from build123d import *

# Parameters (mm, degrees)
SKETCH1_W           = 3.5
SKETCH1_H           = 3.5
BOSS_EXTRUDE1_DEPTH = 1.81
SKETCH2_W           = 0.5
SKETCH2_H           = 0.5
BOSS_EXTRUDE2_DEPTH = 3
SKETCH6_R           = 1
CUT_EXTRUDE1_DEPTH  = 0.001
SKETCH7_R           = 1.2
BOSS_EXTRUDE6_DEPTH = 2.69
HOLE1_D             = 1.6
HOLE1_DEPTH         = 1.45
CHAMFER3_SIZE       = 0.15
SKETCH12_R          = 0.381
BOSS_EXTRUDE7_DEPTH = 3.001
CHAMFER1_SIZE       = 0.15
CHAMFER2_SIZE       = 0.35
CHAMFER2_SIZE2      = 0.15


with BuildPart() as part:
    # Sketch1 → Boss-Extrude1 (new body)
    with BuildSketch(Plane.XZ):
        Rectangle(SKETCH1_W, SKETCH1_H)
    extrude(amount=-BOSS_EXTRUDE1_DEPTH)

    # Sketch2 → Boss-Extrude2 (add)
    with BuildSketch(Plane.XZ):
        with Locations((-1.27, -1.27)):
            Rectangle(SKETCH2_W, SKETCH2_H)
        with Locations((1.27, -1.27)):
            Rectangle(SKETCH2_W, SKETCH2_H)
        with Locations((1.27, 1.27)):
            Rectangle(SKETCH2_W, SKETCH2_H)
        with Locations((-1.27, 1.27)):
            Rectangle(SKETCH2_W, SKETCH2_H)
    extrude(amount=BOSS_EXTRUDE2_DEPTH)

    # Sketch6 → Cut-Extrude1 (cut)
    with BuildSketch(Plane.XZ):
        with Locations(Location((0, 0, 0), (0, 0, 90))):
            Circle(SKETCH6_R)
    extrude(amount=-CUT_EXTRUDE1_DEPTH, mode=Mode.SUBTRACT)

    # Sketch7 → Boss-Extrude6 (add)
    with BuildSketch(Plane(origin=(0, 1.81, 0), x_dir=(-1, 0, 0), z_dir=(0, 1, 0))):
        with Locations(Location((0, 0, 0), (0, 0, 270))):
            Circle(SKETCH7_R)
    extrude(amount=BOSS_EXTRUDE6_DEPTH)

    # Hole1
    with Locations(Plane(origin=(0, 4.5, 0), x_dir=(1, 0, 0), z_dir=(0, 1, 0))):
        with Locations((0, 0)):
            Hole(HOLE1_D / 2, depth=HOLE1_DEPTH)

    # Sketch10 → Revolve1 (revolve)
    with BuildSketch(Plane(origin=(0, 0, 0), x_dir=(-1, 0, 0), z_dir=(0, 0, -1)), mode=Mode.PRIVATE) as revolve1_sk:
        Polygon((-0.19, 3.05), (0, 3.05), (0, 4.37), (-0.0405, 4.37), (-0.19, 4.37), (-0.19, 4.220000833), align=None)
    revolve(revolve1_sk.sketch.rotate(Axis((0, 3.05, 0), (0, 1, 0)), 270), axis=Axis((0, 3.05, 0), (0, 1, 0)))

    # Chamfer3
    chamfer3_edges = [part.edges().sort_by_distance(p)[0] for p in [
        (0, 4.37, -0.19),
    ]]
    chamfer(chamfer3_edges, length=CHAMFER3_SIZE)

    # Sketch12 → Boss-Extrude7 (add)
    with BuildSketch(Plane.XZ.offset(-0.001)):
        with Locations(Location((0, 0, 0), (0, 0, 90))):
            Circle(SKETCH12_R)
    extrude(amount=BOSS_EXTRUDE7_DEPTH)

    # Chamfer1
    chamfer1_edges = [part.edges().sort_by_distance(p)[0] for p in [
        (0, -3, -0.381),
    ]]
    chamfer(chamfer1_edges, length=CHAMFER1_SIZE)

    # Chamfer2
    chamfer2_edges = [part.edges().sort_by_distance(p)[0] for p in [
        (0, 4.5, 1.2),
    ]]
    chamfer2_side = [part.faces().sort_by_distance(p)[0] for p in [
        (0, 3.155, 1.2),
    ]]
    chamfer(chamfer2_edges, length=CHAMFER2_SIZE, length2=CHAMFER2_SIZE2, reference=chamfer2_side[0])


solid = part.part
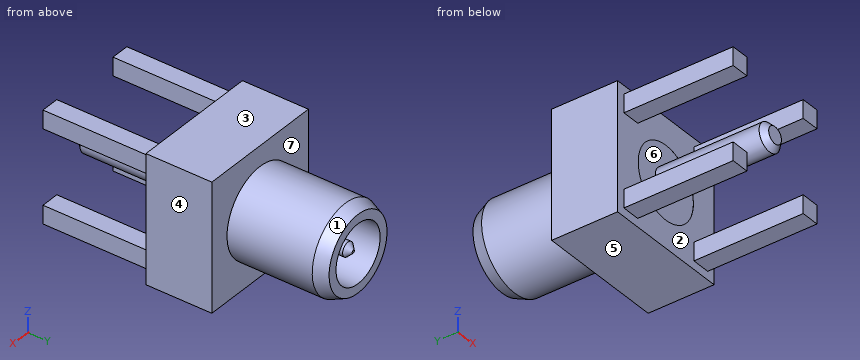
Part model, mm, in its own coordinate system. Face numbers are marked on the shaded views. A direction names the side the tool comes from. Coordinates: 2 decimals unless noted, no trailing zeros. Write each loop counter-clockwise with the first axis right and the second up, starting at its lowest first coordinate (ties: lowest second). Pieces come first, ordered by that corner, then holes. Notation, with made-up numbers: (82.5, 28) - (130.5, 28) arc R25 ccw to (130.5, 65) - close; hole circle Ø9 at (1.5, -24). An arc over 180 degrees is marked (long way). Put each result on its own line as item: value.
1. Probe line 1 along X through (y, z) = (-1.5, 1.4); line 2 along Y through (x, z) = (0.05, 0.65); line 3 along Y through (x, z) = (1.4, 0.45). List the from-to ranges inside material, lowest first. Write a range as [from, to].
Final values:
line 1: x = [-1.52, -1.02], [1.02, 1.52]
line 2: y = [0, 3.05]
line 3: y = [0, 1.81]
2. 3-axis set-ups, long thin cutter, end or side, ignore diameter. For the marked faces 5, 6 and 7: which of +Z, -Z, +X, -X, +Y, -Y reach the whole face in a straight line?
Final values:
face 5: -Z, +X, -X, +Y, -Y
face 6: -Y
face 7: +Y
3. Flat gauge pins, fed straight in: pin 1 Ø0.6 at (x, y) = (-1.5, -1.5) entering from -Z; pin 2 Ø2 at (x, y) = (1, -1.5) entering from +Z; pin 3 Ø0.6 at (y, z) = (-1.5, -1.5) entering from -X. Where does each tip first touch, or does it go through?
Final values:
pin 1: stops at z = -1.52
pin 2: stops at z = 1.52
pin 3: stops at x = -1.52
4. Band-saw the part on B-B (y = -1). Write the cut outline in (x, z), then the cut area to 3 significant figures.
Final values:
outline: (-1.52, -1.52) - (-1.02, -1.52) - (-1.02, -1.02) - (-1.52, -1.02) - close; (-1.52, 1.02) - (-1.02, 1.02) - (-1.02, 1.52) - (-1.52, 1.52) - close; circle Ø0.76 at (0, 0); (1.02, -1.52) - (1.52, -1.52) - (1.52, -1.02) - (1.02, -1.02) - close; (1.02, 1.02) - (1.52, 1.02) - (1.52, 1.52) - (1.02, 1.52) - close
area: 1.46 mm²
5. Band-saw the part on C-C (z = 1.4). Write the cut outline in (x, y), then the cut area to 4 significant figures.
Final values:
outline: (-1.75, 0) - (-1.52, 0) - (-1.52, -3) - (-1.02, -3) - (-1.02, 0) - (1.02, 0) - (1.02, -3) - (1.52, -3) - (1.52, 0) - (1.75, 0) - (1.75, 1.81) - (-1.75, 1.81) - close
area: 9.335 mm²
6. Band-saw the part on D-D (x = 1.3). Write the cut outline in (y, z), then the cut area to 4 significant figures.
Final values:
outline: (-3, -1.52) - (0, -1.52) - (0, -1.75) - (1.81, -1.75) - (1.81, 1.75) - (0, 1.75) - (0, 1.52) - (-3, 1.52) - (-3, 1.02) - (0, 1.02) - (0, -1.02) - (-3, -1.02) - close
area: 9.335 mm²
7. Band-saw the part on A-A (y = 3.25). Write the cut outline in (x, z).
Final values:
outline: circle Ø2.4 at (0, 0); circle Ø0.38 at (0, 0); hole circle Ø1.6 at (0, 0)
8. Two-plate mould, pull along Z, no slides. Class the marked faces 1, 2, 3 and 4: +Z half, -Z half, draft (parallel to the pull), parting line (faces both ways), or undercut.
Final values:
face 1: parting line
face 2: undercut
face 3: +Z half
face 4: draft
